from build123d import *

# Parameters (mm, degrees)
F0_W     = 290
F0_H     = 250
F1_DEPTH = 9
F2_R     = 3.96875
F3_DEPTH = 9
F4_R     = 3.96875
F5_DEPTH = 9


with BuildPart() as f1:
    # F0 (on Top) → F1 (new body, symmetric)
    with BuildSketch(Plane.XY):
        Rectangle(F0_W, F0_H)
    extrude(amount=F1_DEPTH, both=True)

    # F2 (on face) → F3 (cut)
    with BuildSketch(Plane.XY.offset(9)):
        with Locations((136, 0)):
            Circle(F2_R)
        with Locations((136, 96)):
            Circle(F2_R)
        with Locations((136, -96)):
            Circle(F2_R)
    extrude(amount=-F3_DEPTH, mode=Mode.SUBTRACT)

    # F4 (on face) → F5 (cut)
    with BuildSketch(Plane(origin=(-145, 0, 0), x_dir=(0, -1, 0), z_dir=(-1, 0, 0))):
        Circle(F4_R)
        with Locations((96, 0)):
            Circle(F4_R)
        with Locations((-96, 0)):
            Circle(F4_R)
    extrude(amount=-F5_DEPTH, mode=Mode.SUBTRACT)


solid = f1.part
Work out the finished part from the listing and answer in its coordinate system (mm). A direction names the side the tool comes from. Give positions to 0.01 mm unless a question says otherwise; leave off trailing zeros. Loops run counter-clockwise (first coordinate to the right, second up) from the corner with the lowest first, then second, coordinate; pieces in that order, holes last. Notation, with made-up numbers: (67, 34) -> (89, 34) arc R23 ccw to (89, 66) -> close; hole circle Ø4 at (5, 71). An arc over 180 degrees is marked (long way). Use a Markdown table: item, result. Add a question column.
1) The part is cut by section A-A, the plane y = 96. Determine the outline of the cut face in (x, z), plus the area to 3 significant figures.
2) Each of these flat-tipped pins is pushed along its axis until it touches: P1, Ø4, axis at x = 135, y = -1, coming from the +Z side; P2, Ø2.5, axis at y = 95.5, z = -1, coming from the -X side. Where does it stop, or does it pass through?
3) Consider line 1 along Y through (x, z) = (136, 3.75); line 2 along Z through (x, y) = (-142, -96); line 3 along X through (y, z) = (-2, 2.75). Determine where each line is inside the solid, lowest interval first.
4) Which of the six approach directions +Z, -Z, +X, -X, +Y, -Y give full straight-line access (tool end or side, diameter ignored) to faces 1 (the flat face through (-2, -125, 0)), 2 (the flat face through (136, 0, 0)), 3 (the cylindrical face through (-140.563, 92.215, 1.192))?
5) For a pull along X with two mould halves and no side action, classify faces 4 (the flat face through (136, -96, 0)), 5 (the cylindrical face through (-140.563, 0.86, -3.874)), 6 (the flat face through (-136, 0, 0)) as +X half, -X half, draft (parallel to the pull), parting line (faces both ways), or undercut.
Reported:
| question | item | result |
|---|---|---|
| 1 | outline | (-145, -9) -> (145, -9) -> (145, 9) -> (139.97, 9) -> (139.97, 0) -> (132.03, 0) -> (132.03, 9) -> (-145, 9) -> (-145, 3.97) -> (-136, 3.97) -> (-136, -3.97) -> (-145, -3.97) -> close |
| 1 | area | 5,080 mm^2 |
| 2 | P1 | stops at z = 0 |
| 2 | P2 | stops at x = -136 |
| 3 | line 1 | y = -125 to -99.97, -92.03 to -3.97, 3.97 to 92.03, 99.97 to 125 |
| 3 | line 2 | z = -9 to -3.97, 3.97 to 9 |
| 3 | line 3 | x = -136 to 132.57, 139.43 to 145 |
| 4 | face 1 | +Z, -Z, +X, -X, -Y |
| 4 | face 2 | +Z |
| 4 | face 3 | -X |
| 5 | face 4 | undercut |
| 5 | face 5 | draft |
| 5 | face 6 | -X half |
